The listing builds one solid part. Answer for the finished solid, in the listing's coordinates (mm). Face numbers are marked on the shaded views. Coordinates: 2 decimals unless noted, no trailing zeros. Order: outer loops, then holes, each group sorted by start corner. A loop starts at its lowest first (then second) coordinate and runs counter-clockwise, first axis right, second up. Notation, with made-up numbers: (88.5, 77) -> (112.5, 77) arc R25 cw to (112.5, 93) -> close; hole circle Ø10 at (70, 18). An arc over 180 degrees is marked (long way). Return JSON: item names as keys, results as strings.
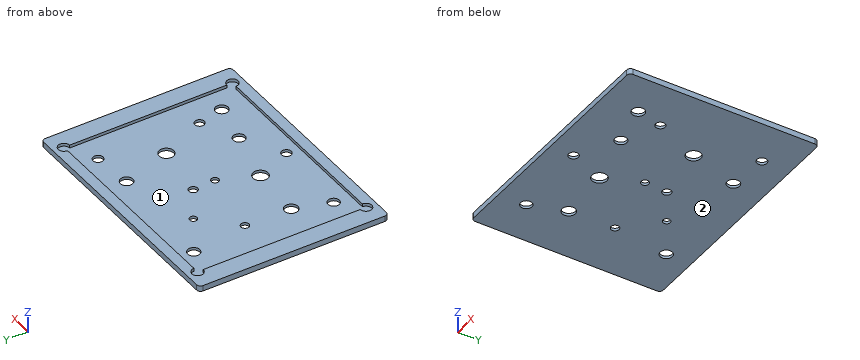
from build123d import *

# Parameters (mm, degrees)
SKETCH_W        = 130
SKETCH_H        = 100
PAD_DEPTH       = 3
POCKET_DEPTH    = 1.6
SKETCH002_R     = 2
SKETCH002_R_2   = 3.501224
SKETCH002_R_3   = 3.145499
SKETCH002_R_4   = 3.838243
SKETCH002_R_5   = 3.281325
SKETCH002_R_6   = 2.288685
SKETCH002_R_7   = 1.945006
SKETCH002_R_8   = 2.13236
SKETCH002_R_9   = 3.927242
SKETCH002_R_10  = 2.558827
SKETCH002_R_11  = 2.9792
SKETCH002_R_12  = 2.479414
SKETCH002_R_13  = 2.648073
SKETCH002_R_14  = 3.212751
SKETCH002_R_15  = 3.309638
POCKET001_DEPTH = 3.001
FILLET_R        = 2


with BuildPart() as part:
    # Sketch → Pad (new body)
    with BuildSketch(Plane.XY):
        with Locations((65, 50)):
            Rectangle(SKETCH_W, SKETCH_H)
    extrude(amount=PAD_DEPTH)

    # Sketch001 (on Face6 of Pad) → Pocket (cut)
    with BuildSketch(Plane.XY.offset(3)):
        with BuildLine():
            ThreePointArc((117, 5.55), (122.12132, 3.42868), (120, 8.55))
            Line((120, 91.45), (120, 8.55))
            ThreePointArc((120, 91.45), (122.12132, 96.57132), (117, 94.45))
            Line((13, 94.45), (117, 94.45))
            ThreePointArc((13, 94.45), (7.87868, 96.57132), (10, 91.45))
            Line((10, 8.55), (10, 91.45))
            ThreePointArc((10, 8.55), (7.87868, 3.42868), (13, 5.55))
            Line((117, 5.55), (13, 5.55))
        make_face()
    extrude(amount=-POCKET_DEPTH, mode=Mode.SUBTRACT)

    # Sketch002 (on Face4 of Pocket) → Pocket001 (cut, through all)
    with BuildSketch(Plane(origin=(0, 0, 0), x_dir=(1, 0, 0), z_dir=(0, 0, -1))):
        with Locations((65, -50)):
            Circle(SKETCH002_R)
        with Locations((28.844851, -32.958813)):
            Circle(SKETCH002_R_2)
        with Locations((85.680542, -23.994795)):
            Circle(SKETCH002_R_3)
        with Locations((93.500214, -57.371456)):
            Circle(SKETCH002_R_4)
        with Locations((85.489815, -83.50061)):
            Circle(SKETCH002_R_5)
        with Locations((64.319481, -61.948826)):
            Circle(SKETCH002_R_6)
        with Locations((46.009991, -73.582977)):
            Circle(SKETCH002_R_7)
        with Locations((29.417021, -56.990009)):
            Circle(SKETCH002_R_8)
        with Locations((57.071968, -31.051573)):
            Circle(SKETCH002_R_9)
        with Locations((64.878792, -12.373779)):
            Circle(SKETCH002_R_10)
        with Locations((22.74169, -14.45861)):
            Circle(SKETCH002_R_11)
        with Locations((104.56218, -32.768085)):
            Circle(SKETCH002_R_12)
        with Locations((106.376934, -85.169306)):
            Circle(SKETCH002_R_13)
        with Locations((25.178326, -86.726067)):
            Circle(SKETCH002_R_14)
        with Locations((107.791985, -19.028767)):
            Circle(SKETCH002_R_15)
    extrude(amount=-POCKET001_DEPTH, mode=Mode.SUBTRACT)

    # Fillet
    fillet_edges = [part.edges().sort_by_distance(p)[0] for p in [
        (130, 0, 1.5),
        (0, 0, 1.5),
        (130, 100, 1.5),
        (0, 100, 1.5),
    ]]
    fillet(fillet_edges, radius=FILLET_R)


solid = part.part
1. Consider line 1 (X direction, y = 16.5, z = 0.65); line 2 (X direction, y = 65, z = 2.55); line 3 (X direction, y = 5, z = 1.9). Determine where each line is inside the solid, lowest interval first. Write a range as from..to.
Answer block:
{"line 1": "x = 0..20.57, 24.91..105.66, 109.93..130", "line 2": "x = 0..10, 120..130", "line 3": "x = 0..7.05, 12.95..117.05, 122.95..130"}
2. The part is cut by section A-A on y = 50. Give the vertices of the cut face in (x, z), and give its area (3 significant figures).
Answer block:
{"outline": "(0, 0) -> (63, 0) -> (63, 1.4) -> (10, 1.4) -> (10, 3) -> (0, 3) -> close; (67, 0) -> (130, 0) -> (130, 3) -> (120, 3) -> (120, 1.4) -> (67, 1.4) -> close", "area": "208 mm2"}
3. The part is cut by section C-C on x = 75.5. Give the vertices of the cut face in (y, z).
Answer block:
{"outline": "(0, 0) -> (100, 0) -> (100, 3) -> (94.45, 3) -> (94.45, 1.4) -> (5.55, 1.4) -> (5.55, 3) -> (0, 3) -> close"}
4. Each of these flat-tipped pins is pushed along its axis until it touches: pin 1 Ø4 at (x, y) = (104.56, 32.77) entering from +Z; pin 2 Ø6.5 at (x, y) = (65, 50) entering from +Z; pin 3 Ø9.5 at (x, y) = (120, 5.55) entering from -Z. Where does it stop, or does it pass through?
Answer block:
{"pin 1": "passes through", "pin 2": "stops at z = 1.4", "pin 3": "stops at z = 0"}
5. The part is cut by section B-B on z = 2.25. Give the vertices of the cut face in (x, y).
Answer block:
{"outline": "(0, 2) arc R2 ccw to (2, 0) -> (128, 0) arc R2 ccw to (130, 2) -> (130, 98) arc R2 ccw to (128, 100) -> (2, 100) arc R2 ccw to (0, 98) -> close; hole (10, 8.55) arc R3 ccw (long way) to (13, 5.55) -> (117, 5.55) arc R3 ccw (long way) to (120, 8.55) -> (120, 91.45) arc R3 ccw (long way) to (117, 94.45) -> (13, 94.45) arc R3 ccw (long way) to (10, 91.45) -> close"}
6. Determine the mould class of the marked faces 1 and 2 for opening direction X: pulls with the +X half, pulls with the -X half, needs draft (parallel to the pull), parting line crosses it, or undercut.
Answer block:
{"face 1": "undercut", "face 2": "needs draft"}
